from build123d import *

# Parameters (mm, degrees)
F1_DEPTH = 25.4


with BuildPart() as f1:
    # F0 (on Top) → F1 (new body)
    with BuildSketch(Plane.XY):
        Polygon((70.085101, 53.899866), (-68.491101, 56.833832), (-78.651101, 56.833832), (-78.651101, -56.953683), (-30.996239, -56.953683), (-30.996239, -19.086355), (-23.3617, -19.086355), (-23.3617, -23.972463), (0, -23.972463), (0, -16.032539), (14.811011, -16.032539), (14.811011, -56.037541), (70.085101, -56.037541), align=None)
        Polygon((-68.491101, -10.769275), (-68.491101, 46.673832), (-2.841839, 46.673832), (26.465869, 46.673832), (61.244347, 46.673832), (61.244347, 15.803046), (61.244347, -10.769275), (61.244347, -49.455448), (20.213559, -49.455448), (20.213559, -10.769275), (-4.014147, -10.769275), (-4.014147, -16.630817), (-18.472611, -16.630817), (-18.472611, -10.769275), (-39.964932, -10.769275), (-39.964932, -48.283138), (-68.491101, -48.283138), align=None, mode=Mode.SUBTRACT)
    extrude(amount=F1_DEPTH)


solid = f1.part
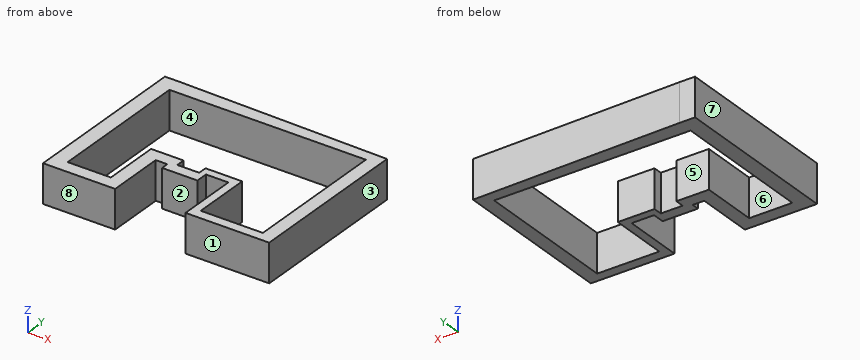
Can you work these out from the model? Positions are in its coordinate system, mm. Face numbers are marked on the shaded views. A direction names the side the tool comes from. Coordinates: 2 decimals unless noted, no trailing zeros. Write each loop counter-clockwise with the first axis right and the second up, starting at its lowest first coordinate (ties: lowest second). Pieces come first, ordered by that corner, then holes. Notation, with made-up numbers: M -4.75,-24.5 L 50.25,-24.5 A10 cw 50.25,-12.5 Z; hole C 15.25,59.5 d7. An arc over 180 degrees is marked long. Use one line per item in the form item = value.
Q1. If we section it at A-A (y = 3): Write out the boundary of the cut face in (x, z), then the cut area to 3 significant figures.
Model answer:
outline = M -78.65,0 L -68.49,0 L -68.49,25.4 L -78.65,25.4 Z; M 61.24,0 L 70.09,0 L 70.09,25.4 L 61.24,25.4 Z
area = 483 mm^2
Q2. For P1, Ø12.5, axis at x = -50.5, z = 15.5, coming from the +Y side; P2, Ø12.5, axis at x = -22, z = 15, coming from the -Y side; P3, Ø6.5, axis at x = -25.5, z = 15, coming from the +Y side, each with a flat end and sliding along its axis, tell me the tip position at first contact or that it passes through.
Model answer:
P1 = 56.59
P2 = -23.97
P3 = 55.99
Q3. For the marked faces 1, 2, 3 and 4, which set-ups out of +Z, -Z, +X, -X, +Y, -Y let a thin tool reach every point of the face, with its end or its side?
Model answer:
face_1 = +Z, -Z, +X, -Y
face_2 = +Z, -Z, -Y
face_3 = +Z, -Z, +X, +Y, -Y
face_4 = +Z, -Z
Q4. We'd pull the mould along X, two halves only. Please class the marked faces 5, 6, 7 and 8: +X half, -X half, draft (parallel to the pull), parting line (faces both ways), or undercut.
Model answer:
face_5 = undercut
face_6 = undercut
face_7 = -X half
face_8 = draft
Q5. I need wall thicknesses on line 1 along X through (y, z) = (-34, 17.5); line 2 along X through (y, z) = (29.5, 13); line 3 along Y through (x, z) = (-68, 5.75). Which ranges of each line are inside material? Lowest first, please. Write a range as from..to.
Model answer:
line_1 = -78.65..-68.49, -39.96..-31, 14.81..20.21, 61.24..70.09
line_2 = -78.65..-68.49, 61.24..70.09
line_3 = -56.95..-48.28, 46.67..56.82
Q6. If we section it at B-B (z = 19.5): Write out the boundary of the cut face in (x, y), then the cut area to 3 significant figures.
Model answer:
outline = M -78.65,-56.95 L -31,-56.95 L -31,-19.09 L -23.36,-19.09 L -23.36,-23.97 L 0,-23.97 L 0,-16.03 L 14.81,-16.03 L 14.81,-56.04 L 70.09,-56.04 L 70.09,53.9 L -68.49,56.83 L -78.65,56.83 Z; hole M -68.49,-48.28 L -39.96,-48.28 L -39.96,-10.77 L -18.47,-10.77 L -18.47,-16.63 L -4.01,-16.63 L -4.01,-10.77 L 20.21,-10.77 L 20.21,-49.46 L 61.24,-49.46 L 61.24,46.67 L -68.49,46.67 Z
area = 4,810 mm^2
Q7. If we section it at D-D (y = -25.5): Write out the boundary of the cut face in (x, z), then the cut area to 3 significant figures.
Model answer:
outline = M -78.65,0 L -68.49,0 L -68.49,25.4 L -78.65,25.4 Z; M -39.96,0 L -31,0 L -31,25.4 L -39.96,25.4 Z; M 14.81,0 L 20.21,0 L 20.21,25.4 L 14.81,25.4 Z; M 61.24,0 L 70.09,0 L 70.09,25.4 L 61.24,25.4 Z
area = 848 mm^2
Q8. If we section it at C-C (x = 23): Write out the boundary of the cut face in (y, z).
Model answer:
outline = M -56.04,0 L -49.46,0 L -49.46,25.4 L -56.04,25.4 Z; M 46.67,0 L 54.9,0 L 54.9,25.4 L 46.67,25.4 Z
